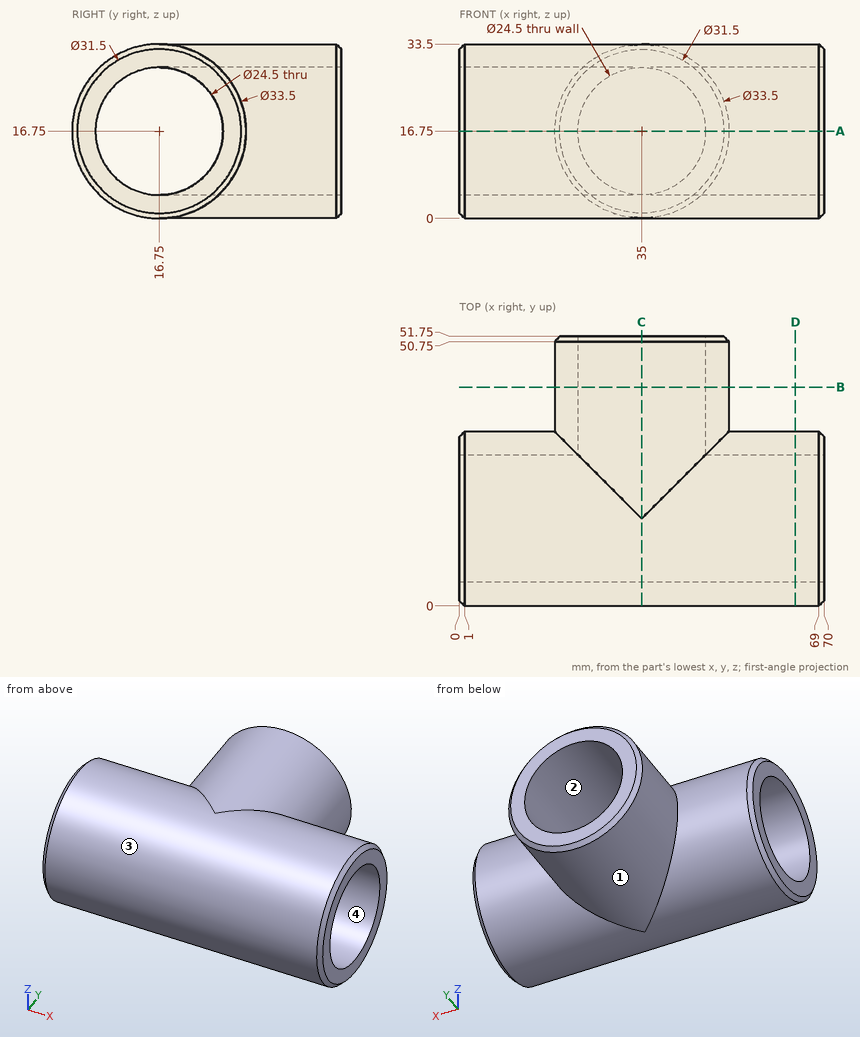
The drawing under review shows one solid part. Ordinate dimensions are in mm from its lowest x, y, z. A direction names the side the tool comes from. Give positions to 0.01 mm unless a question says otherwise; leave off trailing zeros. Order: outer loops, then holes, each group sorted by start corner. A loop starts at its lowest first (then second) coordinate and runs counter-clockwise, first axis right, second up. Notation, with made-up numbers: (-19, 46.25) -> (34, 46.25) arc R34 cw to (34, 81.25) -> close; hole circle Ø5 at (-6.75, 23.5). An arc over 180 degrees is marked (long way). Write item = value, one per line.
1) For the marked faces 3 and 4, list the 3-axis set-ups (+Z, -Z, +X, -X, +Y, -Y) from which the entire face can be reached by the end or side of a thin tool; tool diameter is ignored.
Findings:
face_3 = none
face_4 = +X, -X
2) We need section B-B, the plane y = 42. Give the boundary of the cut face in (x, z).
Findings:
outline = circle Ø33.5 at (35, 16.75); hole circle Ø24.5 at (35, 16.75)
3) We need section A-A, the plane z = 16.75. Give the boundary of the cut face in (x, y).
Findings:
outline = (0, 1) -> (1, 0) -> (69, 0) -> (70, 1) -> (70, 4.5) -> (0, 4.5) -> close; (0, 29) -> (22.75, 29) -> (22.75, 51.75) -> (19.25, 51.75) -> (18.25, 50.75) -> (18.25, 33.5) -> (1, 33.5) -> (0, 32.5) -> close; (47.25, 29) -> (70, 29) -> (70, 32.5) -> (69, 33.5) -> (51.75, 33.5) -> (51.75, 50.75) -> (50.75, 51.75) -> (47.25, 51.75) -> close
4) We need section C-C, the plane x = 35. Give the boundary of the cut face in (y, z), and give its area (3 significant figures).
Findings:
outline = (16.75, 0) -> (50.75, 0) -> (51.75, 1) -> (51.75, 4.5) -> (16.75, 4.5) arc R12.25 cw to (16.75, 29) -> (51.75, 29) -> (51.75, 32.5) -> (50.75, 33.5) -> (16.75, 33.5) arc R16.75 ccw to start
area = 519 mm^2
5) We need section D-D, the plane x = 64.5. Give the boundary of the cut face in (y, z), and give its area (3 significant figures).
Findings:
outline = circle Ø33.5 at (16.75, 16.75); hole circle Ø24.5 at (16.75, 16.75)
area = 410 mm^2
6) Insertion check: pin 1 (2 mm diameter, centred on y = 44, z = 11, fed in from -X); pin 2 (12 mm diameter, centred on y = 46, z = 26.5, fed in from -X); pin 3 (2 mm diameter, centred on x = 47.5, y = 38, fed in from +Z). Each pin has a flat end and moves straight along its axis. Give the tip position at first contact, or say it passes through.
Findings:
pin_1 = 18.94
pin_2 = 18.68
pin_3 = 28.93
7) Draft analysis for pull direction X (two halves, no side actions). For the marked faces 1 and 2, state which applies: pulls with the +X half, pulls with the -X half, needs draft (parallel to the pull), parting line crosses it, or undercut.
Findings:
face_1 = parting line crosses it
face_2 = undercut
8) To check wall thickness, follow L1, parallel to Z at x = 56.5, y = 16.75; L2, parallel to X at y = 40, z = 16.75; L3, parallel to X at y = 35.5, z = 12. State the ranges of each line that lie inside material, in increasing order. Write a range as from..to.
Findings:
L1 = 0..4.5, 29..33.5
L2 = 18.25..22.75, 47.25..51.75
L3 = 18.94..23.71, 46.29..51.06
